from build123d import *

# Parameters (mm, degrees)
F1_DEPTH  = 48.514
F2_R      = 3.175
F3_DEPTH  = 19.558
F4_R      = 3.175
F5_DEPTH  = 19.685
F6_R      = 26.9875
F7_DEPTH  = 8.6995
F9_R      = 5.55625
F10_DEPTH = 2.921


with BuildPart() as f1:
    # F0 (on Front) → F1 (new body, symmetric)
    with BuildSketch(Plane.XZ):
        with BuildLine():
            ThreePointArc((9.779, 16.0655), (9.407026, 16.963526), (8.509, 17.3355))
            Line((8.509, 17.3355), (-8.509, 17.3355))
            ThreePointArc((-8.509, 17.3355), (-9.407026, 16.963526), (-9.779, 16.0655))
            Line((-9.779, 16.0655), (-9.779, -17.3355))
            Line((-9.779, -17.3355), (-6.858, -17.3355))
            Line((-6.858, -17.3355), (-6.858, 13.1445))
            ThreePointArc((-6.858, 13.1445), (-6.486026, 14.042526), (-5.588, 14.4145))
            Line((-5.588, 14.4145), (5.588, 14.4145))
            ThreePointArc((5.588, 14.4145), (6.486026, 14.042526), (6.858, 13.1445))
            Line((6.858, 13.1445), (6.858, -17.3355))
            Line((6.858, -17.3355), (9.779, -17.3355))
            Line((9.779, -17.3355), (9.779, 16.0655))
        make_face()
    extrude(amount=F1_DEPTH, both=True)

    # F2 (on face) → F3 (cut, through all)
    with BuildSketch(Plane.YZ.offset(9.779)):
        with Locations((-31.75, -3.6195)):
            Circle(F2_R)
        with Locations((31.75, -3.6195)):
            Circle(F2_R)
    extrude(amount=-F3_DEPTH, mode=Mode.SUBTRACT)

    # F4 (on Right) → F5 (join, symmetric)
    with BuildSketch(Plane.YZ):
        with Locations((-31.75, -3.6195)):
            Circle(F4_R)
        with Locations((31.75, -3.6195)):
            Circle(F4_R)
    extrude(amount=F5_DEPTH, both=True)

    # F6 (on face) → F7 (join)
    with BuildSketch(Plane.YZ.offset(19.685)):
        with Locations((-31.75, -3.6195)):
            Circle(F6_R)
        with Locations((31.75, -3.6195)):
            Circle(F6_R)
    extrude(amount=-F7_DEPTH)

    # F8: F1 across plane


with BuildPart() as f1_1:
    add(f1.part)
    add(f1.part.mirror(Plane.YZ))

    # F9 (on face) → F10 (cut, through all)
    with BuildSketch(Plane.XY.offset(17.3355)):
        Circle(F9_R)
    extrude(amount=-F10_DEPTH, mode=Mode.SUBTRACT)


solid = f1_1.part
Source: CAD feature listing. Evaluate the final solid. Frame: model axes, mm. A direction names the side the tool comes from. Round coordinates to 2 decimals unless told otherwise and drop trailing zeros. Order: outer loops, then holes, each group sorted by start corner. A loop starts at its lowest first (then second) coordinate and runs counter-clockwise, first axis right, second up. Notation, with made-up numbers: (14.5, 19) - (65.5, 19) arc R21 cw to (65.5, 23) - close; hole circle Ø11 at (33.5, 6.5). An arc over 180 degrees is marked (long way). Use a Markdown table: item, result. Add a question column.
1. Section query C-C (z = 5). Return the cut outline in (x, y) (1 decimal), then the cut area to 3 significant figures.
2. Mould query, pull axis Z, two halves, no side actions, for faces 1 (the flat face through (-19.685, -32, -3)), 2 (the cylindrical face through (15.4, 56.68, -13.96)), 3 (the cylindrical face through (0.1, 31.06, -6.72)). Classes: +Z half, -Z half, draft (parallel to the pull), parting line (faces both ways), or undercut.
3. Set-up query: faces 4 (the cylindrical face through (15.4, -53.2, -20)), 5 (the cylindrical face through (10.37, -34.92, -3.48)), 6 (the cylindrical face through (-15.4, 56.68, -13.96)), 7 (the flat face through (8, -1, -17.336)), 8 (the flat face through (0, -11, 14.414)). Return all of +Z, -Z, +X, -X, +Y, -Y with unobstructed straight access to the full face (end or side cutting, diameter ignored); none if empty.
4. Section query D-D (x = 2.5). Give the number of separate pieces and of enclosed holes in the cut face, then the cut area to 3 significant figures.
5. First-contact query: pin 1 (4 mm diameter, centred on x = -7.5, z = -17, fed in from -Y); pin 2 (18 mm diameter, centred on x = 0, y = 0, fed in from -Z); pin 3 (2 mm diameter, centred on x = -8.5, z = -21, fed in from -Y); pin 4 (18.5 mm diameter, centred on x = -2, y = -11, fed in from +Z). Flat tips, straight axial feed; report the tip coordinate or a pass-through.
6. Line query: probe 1 along X at (y, z) = (26, 10) (1 decimal); probe 2 along X at (y, z) = (-45, 14) (1 decimal); probe 3 along Y at (x, z) = (0, 16). Output: solid intervals per line, ascending.
Derived:
| question | item | result |
|---|---|---|
| 1 | outline | (-19.7, -57.3) - (-11, -57.3) - (-11, -6.2) - (-19.7, -6.2) - close; (-19.7, 6.2) - (-11, 6.2) - (-11, 57.3) - (-19.7, 57.3) - close; (-9.8, -48.5) - (-6.9, -48.5) - (-6.9, 48.5) - (-9.8, 48.5) - close; (6.9, -48.5) - (9.8, -48.5) - (9.8, 48.5) - (6.9, 48.5) - close; (11, -57.3) - (19.7, -57.3) - (19.7, -6.2) - (11, -6.2) - close; (11, 6.2) - (19.7, 6.2) - (19.7, 57.3) - (11, 57.3) - close |
| 1 | area | 2,350 mm2 |
| 2 | face 1 | draft |
| 2 | face 2 | parting line |
| 2 | face 3 | undercut |
| 3 | face 4 | +X |
| 3 | face 5 | none |
| 3 | face 6 | -X |
| 3 | face 7 | -Z, +Y, -Y |
| 3 | face 8 | +Y, -Y |
| 4 | separate pieces | 4 |
| 4 | enclosed holes | 0 |
| 4 | area | 318 mm2 |
| 5 | pin 1 | y = -48.51 |
| 5 | pin 2 | z = -17.34 |
| 5 | pin 3 | through |
| 5 | pin 4 | z = 17.34 |
| 6 | probe 1 | -19.7 to -11, -9.8 to -6.9, 6.9 to 9.8, 11 to 19.7 |
| 6 | probe 2 | -19.7 to -11, -9.8 to -6.5, 6.5 to 9.8, 11 to 19.7 |
| 6 | probe 3 | -48.51 to -5.56, 5.56 to 48.51 |
